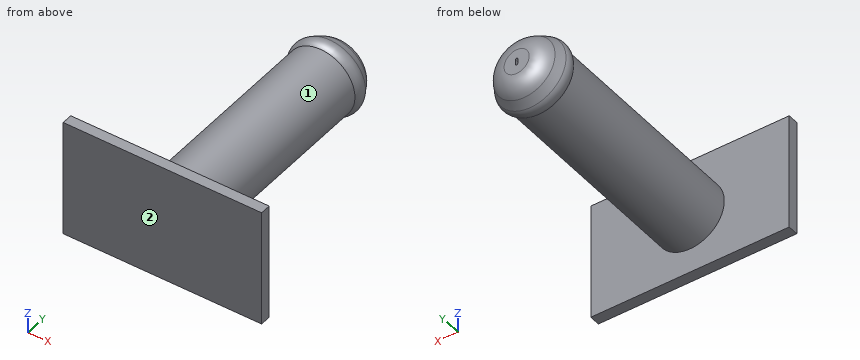
from build123d import *

# Parameters (mm, degrees)
SKETCH2_R           = 32.411320863
BOSS_EXTRUDE1_DEPTH = 200
SKETCH3_R           = 40.764441706
BOSS_EXTRUDE2_DEPTH = 30
BOSS_EXTRUDE2_TAPER = 30
FILLET1_R           = 10
FILLET2_R           = 20
CUT_EXTRUDE1_DEPTH  = 10
SKETCH5_W           = 187.852552736
SKETCH5_H           = 111.255195094
BOSS_EXTRUDE3_DEPTH = 10


with BuildPart() as part:
    # Sketch2 → Boss-Extrude1 (new body)
    with BuildSketch(Plane(origin=(0, 0, 0), x_dir=(1, 0, 0), z_dir=(0, 1, 0))):
        with Locations(Location((0, 0, 0), (0, 0, 270))):
            Circle(SKETCH2_R)
    extrude(amount=BOSS_EXTRUDE1_DEPTH)

    # Sketch3 → Boss-Extrude2 (add)
    with BuildSketch(Plane(origin=(0, 200, 0), x_dir=(1, 0, 0), z_dir=(0, 1, 0))):
        Circle(SKETCH3_R)
    extrude(amount=BOSS_EXTRUDE2_DEPTH, taper=BOSS_EXTRUDE2_TAPER)

    # Fillet1
    # the kernel refuses this fillet: 10 mm, written as the material it takes off along each edge
    with BuildSketch(Plane(origin=(0, 200, 0), x_dir=(1, 0, 0), z_dir=(0, 0, 1))) as fillet1_piece_1:
        with BuildLine():
            CenterArc((25.210979619, 6.93938657), FILLET1_R, 316.057297886, 73.942702114)
            Line((32.411320863, 0), (32.555327688, -0.138787731))
            ThreePointArc((32.555327688, -0.138787731), (36.587881285, -0.2), (40.764441706, -0.2))
            Line((40.764441706, -0.2), (40.937646787, 0.1))
            Line((40.937646787, 0.1), (34.044438737, 12.03938657))
            Line((34.044438737, 12.03938657), (33.871233656, 11.93938657))
        make_face()
    revolve(axis=Axis((0, 200, 0), (0, 1, 0)), mode=Mode.SUBTRACT)

    # Fillet2
    fillet2_edges = [part.edges().sort_by_distance(p)[0] for p in [
        (-23.443933631, 230, 0),
    ]]
    fillet(fillet2_edges, radius=FILLET2_R)

    # Sketch4 → Cut-Extrude1 (cut)
    with BuildSketch(Plane(origin=(0, 230, 0), x_dir=(1, 0, 0), z_dir=(0, 1, 0))):
        with BuildLine():
            Line((1.070724985, 2.258315279), (1.070724985, -2.258315279))
            ThreePointArc((1.070724985, -2.258315279), (0, -3.329040264), (-1.070724985, -2.258315279))
            Line((-1.070724985, -2.258315279), (-1.070724985, 2.258315279))
            ThreePointArc((-1.070724985, 2.258315279), (0, 3.329040264), (1.070724985, 2.258315279))
        make_face()
    extrude(amount=-CUT_EXTRUDE1_DEPTH, mode=Mode.SUBTRACT)

    # Sketch5 → Boss-Extrude3 (add)
    with BuildSketch(Plane.XZ):
        Rectangle(SKETCH5_W, SKETCH5_H)
    extrude(amount=BOSS_EXTRUDE3_DEPTH)


solid = part.part
Geometry: final body of the model. Coordinates: model frame, mm. Face numbers are marked on the shaded views. Give positions to 0.01 mm unless a question says otherwise; leave off trailing zeros. Write each loop counter-clockwise with the first axis right and the second up, starting at its lowest first coordinate (ties: lowest second). Pieces come first, ordered by that corner, then holes. Notation, with made-up numbers: (65.25, 74.25) -> (108.25, 74.25) arc R34 cw to (108.25, 105.25) -> close; hole circle Ø2 at (79.5, 51.5). An arc over 180 degrees is marked (long way). Answer as a JSON object with one key per item and string values.
1. Mould query, pull axis Y, two halves, no side actions, for the marked faces 1 and 2. Classes: pulls with the +Y half, pulls with the -Y half, needs draft (parallel to the pull), parting line crosses it, or undercut.
Ans:
{"face 1": "undercut", "face 2": "pulls with the -Y half"}
2. Contact query for flat-ended pins moving along their axis: pin 1 (2.5 mm diameter, centred on y = 224, z = -0.5, fed in from -X); pin 2 (4 mm diameter, centred on y = 83, z = -36, fed in from -X); pin 3 (6 mm diameter, centred on x = -7.5, y = 178, fed in from -Z); pin 4 (5 mm diameter, centred on y = 226, z = 0, fed in from +X). Output: stop coordinate, or through.
Ans:
{"pin 1": "stops at x = -27.3", "pin 2": "passes through", "pin 3": "stops at z = -32.1", "pin 4": "stops at x = 26.65"}
3. Cut plane D-D on y = 204.5. Output: boundary loops of the cut face in (x, z).
Ans:
{"outline": "circle Ø69.82 at (0, 0)"}
4. Cut plane A-A on x = -49.5. Output: boundary loops of the cut face in (y, z).
Ans:
{"outline": "(-10, -55.63) -> (0, -55.63) -> (0, 55.63) -> (-10, 55.63) -> close"}
5. Ray query, probe 1 along Y at (x, z) = (-57.5, 43); probe 2 along Z at (x, y) = (-6.5, 16.5); probe 3 along X at (y, z) = (217, -12). Return the intervals inside material, ascending. Write a range as from..to.
Ans:
{"probe 1": "y = -10..0", "probe 2": "z = -31.75..31.75", "probe 3": "x = -28.53..28.53"}
6. Cut plane C-C on y = 103. Output: boundary loops of the cut face in (x, z).
Ans:
{"outline": "circle Ø64.82 at (0, 0)"}
7. Cut plane B-B on z = -42. Output: boundary loops of the cut face in (x, y).
Ans:
{"outline": "(-93.93, -10) -> (93.93, -10) -> (93.93, 0) -> (-93.93, 0) -> close"}
